Autodesk Inventor part; units mm, degrees
ref_plane "YZ Plane" through (0, 0, 0) normal (1, 0, 0) x (0, 1, 0)
ref_plane "XZ Plane" through (0, 0, 0) normal (0, 1, 0) x (-1, 0, 0)
ref_plane "XY Plane" through (0, 0, 0) normal (0, 0, 1) x (1, 0, 0)
sketch "Sketch1" plane through (0, 0, 0) normal (0, 1, 0) x (-1, 0, 0)
  circle A0 centre (0, 0) radius 1.5
  dimension "d0" = 3
extrude "Extrusion1" add sketch "Sketch1" along normal blind 34
sketch "Sketch2" plane through (0, 34, 0) normal (0, 1, 0) x (1, 0, 0)
  circle A0 centre (0, 0) radius 1.25
  dimension "d3" = 2.5
extrude "Extrusion2" add sketch "Sketch2" along normal blind 10
thread "Thread1"
fillet "Fillet1" radius 1.25 1 edges at (-1.25, 44, 0)
properties material "Stainless Steel"
Read the model definition and answer for the solid it produces. Units are mm, in the model's axes. A direction names the side the tool comes from. Give positions to 0.01 mm unless a question says otherwise; leave off trailing zeros. Write each loop counter-clockwise with the first axis right and the second up, starting at its lowest first coordinate (ties: lowest second). Pieces come first, ordered by that corner, then holes. Notation, with made-up numbers: (82, 83.5) - (110, 83.5) arc R18 ccw to (110, 113.5) - close; hole circle Ø9 at (37, 75). An arc over 180 degrees is marked (long way). Use CSV: the item, a comma, the result in double quotes. Start each with the question number.
Item 1: The part is cut by section A-A, the plane z = 0. Give the vertices of the cut face in (x, y), and give its area (3 significant figures).
Item 2: The part is cut by section B-B, the plane x = 0. Give the vertices of the cut face in (y, z).
Item 3: The part is cut by section C-C, the plane y = 35.5. Give the vertices of the cut face in (x, z), and give its area (3 significant figures).
Item 4: For faces 1 (the cylindrical face through (-0.27, 38.31, -1.22)), 2 (the cylindrical face through (1.5, 16.76, -0.07)), determine the directions among +Z, -Z, +X, -X, +Y, -Y from which every point of the face is accessible in a straight line to the end or side of a thin tool.
Item 5: A flat-ended cylindrical pin translates along its axis: P1, Ø1.5, axis at x = 1, z = 1, coming from the +Y side. Find the tip coordinate at first contact, or state that the pin passes through.
Item 6: Consider line 1 (Z direction, x = -0.1, y = 8); line 2 (Y direction, x = 0.8, z = 1.15); line 3 (Y direction, x = 1, z = -0.5). Determine where each line is inside the solid, lowest interval first.
Taken from the geometry:
1,outline,"(-1.5, 0) - (1.5, 0) - (1.5, 34) - (1.25, 34) - (1.25, 42.75) arc R1.25 ccw to (-1.25, 42.75) - (-1.25, 34) - (-1.5, 34) - close"
1,area,"126 mm2"
2,outline,"(0, -1.5) - (34, -1.5) - (34, -1.25) - (42.75, -1.25) arc R1.25 ccw to (42.75, 1.25) - (34, 1.25) - (34, 1.5) - (0, 1.5) - close"
3,outline,"circle Ø2.5 at (0, 0)"
3,area,"4.91 mm2"
4,face 1,"+Y"
4,face 2,"+Y, -Y"
5,P1,"y = 43.81"
6,line 1,"-1.5 to 1.5"
6,line 2,"0 to 34"
6,line 3,"0 to 43.31"
